from build123d import *

# Parameters (mm, degrees)
SKETCH1_R           = 2.5
BOSS_EXTRUDE1_DEPTH = 5
FILLET1_R           = 0.5


with BuildPart() as part:
    # Sketch1 → Boss-Extrude1 (new body)
    with BuildSketch(Plane(origin=(0, 0, 0), x_dir=(1, 0, 0), z_dir=(0, 1, 0))):
        Polygon((0, 5), (-4.330127019, 2.5), (-4.330127019, -2.5), (0, -5), (4.330127019, -2.5), (4.330127019, 2.5), align=None)
        with Locations(Location((0, 0, 0), (0, 0, 270))):
            Circle(SKETCH1_R, mode=Mode.SUBTRACT)
    extrude(amount=BOSS_EXTRUDE1_DEPTH)

    # Fillet1
    fillet1_edges = [part.edges().sort_by_distance(p)[0] for p in [
        (-4.330127019, 5, 0),
        (-2.165063509, 5, 3.75),
        (2.165063509, 5, 3.75),
        (0, 5, -2.5),
        (4.330127019, 5, 0),
        (2.165063509, 5, -3.75),
        (-2.165063509, 5, -3.75),
    ]]
    fillet(fillet1_edges, radius=FILLET1_R)


solid = part.part
Could you check a few things on this model? Use its own coordinates, in mm. Round coordinates to 2 decimals unless told otherwise and drop trailing zeros. Write each loop counter-clockwise with the first axis right and the second up, starting at its lowest first coordinate (ties: lowest second). Pieces come first, ordered by that corner, then holes. Notation, with made-up numbers: (13, -20.75) -> (36, -20.75) arc R25 ccw to (36, 17.25) -> close; hole circle Ø4 at (0, 7). An arc over 180 degrees is marked (long way). Use a Markdown table: item, result.
1. Please list where these lines run through material, in increasing order: probe 1 along X at (y, z) = (1.95, 0); probe 2 along Z at (x, y) = (-1.75, 1.2); probe 3 along Z at (x, y) = (-1, 0.85).
Answer key:
| item | result |
|---|---|
| probe 1 | x = -4.33 to -2.5, 2.5 to 4.33 |
| probe 2 | z = -3.99 to -1.79, 1.79 to 3.99 |
| probe 3 | z = -4.42 to -2.29, 2.29 to 4.42 |
2. We'd pull the mould along Z, two halves only. Please class faces 1 (the face through (-2.13, 2.22, -3.77)), 2 (the face through (-4.33, 2, 0)), 3 (the face through (-2.44, 2.22, -0.54)), 4 (the face through (-2.2, 2.22, 3.73)): +Z half, -Z half, draft (parallel to the pull), parting line (faces both ways), or undercut.
Answer key:
| item | result |
|---|---|
| face 1 | -Z half |
| face 2 | draft |
| face 3 | undercut |
| face 4 | +Z half |
3. If we section it at A-A (z = 0): List the corners of the cut face in (x, y) for me, then the cut area to 3 significant figures.
Answer key:
| item | result |
|---|---|
| outline | (-4.33, 0) -> (-2.5, 0) -> (-2.5, 4.5) arc R0.5 ccw to (-3, 5) -> (-3.83, 5) arc R0.5 ccw to (-4.33, 4.5) -> close; (2.5, 0) -> (4.33, 0) -> (4.33, 4.5) arc R0.5 ccw to (3.83, 5) -> (3, 5) arc R0.5 ccw to (2.5, 4.5) -> close |
| area | 18.1 mm^2 |
4. For pin 1 Ø5 at (x, z) = (2.5, -2) entering from -Y; pin 2 Ø2 at (x, y) = (3, 1.5) entering from -Z, each with a flat end and sliding along its axis, tell me the tip position at first contact or that it passes through.
Answer key:
| item | result |
|---|---|
| pin 1 | stops at y = 0 |
| pin 2 | stops at z = -3.85 |
5. If we section it at B-B (y = 3.6): List the corners of the cut face in (x, z) for me.
Answer key:
| item | result |
|---|---|
| outline | (-4.33, -2.5) -> (0, -5) -> (4.33, -2.5) -> (4.33, 2.5) -> (0, 5) -> (-4.33, 2.5) -> close; hole circle Ø5 at (0, 0) |
